from build123d import *

# Parameters (mm, degrees)
F1_DEPTH       = 25
F2_DEPTH       = 10
F3_DEPTH       = 30
F4_DEPTH       = 20
F5_DEPTH       = 10
F7_D           = 14.75
F7_CBORE_D     = 22.25
F7_CBORE_DEPTH = 14
F8_SIZE        = 5
F9_R           = 7.49999


# Not quite as in the source:
# - a fillet or chamfer is up to 0.001 mm smaller than in the source, because OpenCascade refuses the exact size


with BuildPart() as f1:
    # F0 (on Front) → F1 (new body)
    with BuildSketch(Plane.XZ):
        with BuildLine():
            Line((96.5, 100), (-96.5, 100))
            ThreePointArc((-96.5, 100), (-103.5710678119, 97.0710678119), (-106.5, 90))
            Line((-106.5, 90), (-106.5, -90))
            ThreePointArc((-106.5, -90), (-103.5710678119, -97.0710678119), (-96.5, -100))
            Line((-96.5, -100), (-63.5, -100))
            Line((-63.5, -100), (-63.5, -42.2497216032))
            ThreePointArc((-63.5, -42.2497216032), (-58.0047374401, -26.6111405489), (-43.9347826087, -17.8476082112))
            ThreePointArc((-43.9347826087, -17.8476082112), (0.1396103068, 6.3603896932), (24.3476082112, 50.4347826087))
            ThreePointArc((24.3476082112, 50.4347826087), (33.1111405489, 64.5047374401), (48.7497216032, 70))
            Line((48.7497216032, 70), (106.5, 70))
            Line((106.5, 70), (106.5, 90))
            ThreePointArc((106.5, 90), (103.5710678119, 97.0710678119), (96.5, 100))
        make_face()
        with BuildLine():
            ThreePointArc((17.5, 70), (-6.2243507239, 12.7243507239), (-63.5, -11))
            Line((-63.5, -11), (-87.5, -11))
            ThreePointArc((-87.5, -11), (-94.5710678119, -8.0710678119), (-97.5, -1))
            Line((-97.5, -1), (-97.5, 81))
            ThreePointArc((-97.5, 81), (-94.5710678119, 88.0710678119), (-87.5, 91))
            Line((-87.5, 91), (7.5, 91))
            ThreePointArc((7.5, 91), (14.5710678119, 88.0710678119), (17.5, 81))
            Line((17.5, 81), (17.5, 70))
        make_face(mode=Mode.SUBTRACT)
        with BuildLine():
            Line((106.5, 55), (106.5, 70))
            Line((106.5, 70), (48.7497216032, 70))
            ThreePointArc((48.7497216032, 70), (33.1111405489, 64.5047374401), (24.3476082112, 50.4347826087))
            ThreePointArc((24.3476082112, 50.4347826087), (0.1396103068, 6.3603896932), (-43.9347826087, -17.8476082112))
            ThreePointArc((-43.9347826087, -17.8476082112), (-58.0047374401, -26.6111405489), (-63.5, -42.2497216032))
            Line((-63.5, -42.2497216032), (-63.5, -100))
            Line((-63.5, -100), (-48.5, -100))
            Line((-48.5, -100), (-48.5, -42.2497216032))
            ThreePointArc((-48.5, -42.2497216032), (-46.3018949761, -35.9942891815), (-40.6739130435, -32.4888762464))
            ThreePointArc((-40.6739130435, -32.4888762464), (10.7462120246, -4.2462120246), (38.9888762464, 47.1739130435))
            ThreePointArc((38.9888762464, 47.1739130435), (42.4942891815, 52.8018949761), (48.7497216032, 55))
            Line((48.7497216032, 55), (106.5, 55))
        make_face()
        with BuildLine():
            Line((106.5, -40), (106.5, 55))
            Line((106.5, 55), (48.7497216032, 55))
            ThreePointArc((48.7497216032, 55), (42.4942891815, 52.8018949761), (38.9888762464, 47.1739130435))
            ThreePointArc((38.9888762464, 47.1739130435), (10.7462120246, -4.2462120246), (-40.6739130435, -32.4888762464))
            ThreePointArc((-40.6739130435, -32.4888762464), (-46.3018949761, -35.9942891815), (-48.5, -42.2497216032))
            Line((-48.5, -42.2497216032), (-48.5, -100))
            Line((-48.5, -100), (46.5, -100))
            Line((46.5, -100), (46.5, -55))
            ThreePointArc((46.5, -55), (50.8933982822, -44.3933982822), (61.5, -40))
            Line((61.5, -40), (106.5, -40))
        make_face()
        with BuildLine():
            ThreePointArc((46.130896205, 38.7419354839), (49.7234965193, 43.981834214), (55.7476414861, 46))
            Line((55.7476414861, 46), (87.5, 46))
            ThreePointArc((87.5, 46), (94.5710678119, 43.0710678119), (97.5, 36))
            Line((97.5, 36), (97.5, -21))
            ThreePointArc((97.5, -21), (94.5710678119, -28.0710678119), (87.5, -31))
            Line((87.5, -31), (61.5, -31))
            ThreePointArc((61.5, -31), (44.5294372515, -38.0294372515), (37.5, -55))
            Line((37.5, -55), (37.5, -81))
            ThreePointArc((37.5, -81), (34.5710678119, -88.0710678119), (27.5, -91))
            Line((27.5, -91), (-29.5, -91))
            ThreePointArc((-29.5, -91), (-36.5710678119, -88.0710678119), (-39.5, -81))
            Line((-39.5, -81), (-39.5, -49.2476414861))
            ThreePointArc((-39.5, -49.2476414861), (-37.481834214, -43.2234965193), (-32.2419354839, -39.630896205))
            ThreePointArc((-32.2419354839, -39.630896205), (17.1101730553, -10.6101730553), (46.130896205, 38.7419354839))
        make_face(mode=Mode.SUBTRACT)
        with BuildLine():
            Line((106.5, -90), (106.5, -40))
            Line((106.5, -40), (61.5, -40))
            ThreePointArc((61.5, -40), (50.8933982822, -44.3933982822), (46.5, -55))
            Line((46.5, -55), (46.5, -100))
            Line((46.5, -100), (96.5, -100))
            ThreePointArc((96.5, -100), (103.5710678119, -97.0710678119), (106.5, -90))
        make_face()
        with BuildLine():
            Line((-87.5, -11), (-63.5, -11))
            ThreePointArc((-63.5, -11), (-6.2243507239, 12.7243507239), (17.5, 70))
            Line((17.5, 70), (17.5, 81))
            ThreePointArc((17.5, 81), (14.5710678119, 88.0710678119), (7.5, 91))
            Line((7.5, 91), (-87.5, 91))
            ThreePointArc((-87.5, 91), (-94.5710678119, 88.0710678119), (-97.5, 81))
            Line((-97.5, 81), (-97.5, -1))
            ThreePointArc((-97.5, -1), (-94.5710678119, -8.0710678119), (-87.5, -11))
        make_face()
        with BuildLine():
            Line((87.5, 46), (55.7476414861, 46))
            ThreePointArc((55.7476414861, 46), (49.7234965193, 43.981834214), (46.130896205, 38.7419354839))
            ThreePointArc((46.130896205, 38.7419354839), (17.1101730553, -10.6101730553), (-32.2419354839, -39.630896205))
            ThreePointArc((-32.2419354839, -39.630896205), (-37.481834214, -43.2234965193), (-39.5, -49.2476414861))
            Line((-39.5, -49.2476414861), (-39.5, -81))
            ThreePointArc((-39.5, -81), (-36.5710678119, -88.0710678119), (-29.5, -91))
            Line((-29.5, -91), (27.5, -91))
            ThreePointArc((27.5, -91), (34.5710678119, -88.0710678119), (37.5, -81))
            Line((37.5, -81), (37.5, -55))
            ThreePointArc((37.5, -55), (44.5294372515, -38.0294372515), (61.5, -31))
            Line((61.5, -31), (87.5, -31))
            ThreePointArc((87.5, -31), (94.5710678119, -28.0710678119), (97.5, -21))
            Line((97.5, -21), (97.5, 36))
            ThreePointArc((97.5, 36), (94.5710678119, 43.0710678119), (87.5, 46))
        make_face()
    extrude(amount=-F1_DEPTH)

    # F0 (on Front) → F2 (join)
    with BuildSketch(Plane.XZ):
        with BuildLine():
            Line((-87.5, -11), (-63.5, -11))
            ThreePointArc((-63.5, -11), (-6.2243507239, 12.7243507239), (17.5, 70))
            Line((17.5, 70), (17.5, 81))
            ThreePointArc((17.5, 81), (14.5710678119, 88.0710678119), (7.5, 91))
            Line((7.5, 91), (-87.5, 91))
            ThreePointArc((-87.5, 91), (-94.5710678119, 88.0710678119), (-97.5, 81))
            Line((-97.5, 81), (-97.5, -1))
            ThreePointArc((-97.5, -1), (-94.5710678119, -8.0710678119), (-87.5, -11))
        make_face()
    extrude(amount=F2_DEPTH)

    # F0 (on Front) → F3 (join)
    with BuildSketch(Plane.XZ):
        with BuildLine():
            Line((106.5, 55), (106.5, 70))
            Line((106.5, 70), (48.7497216032, 70))
            ThreePointArc((48.7497216032, 70), (33.1111405489, 64.5047374401), (24.3476082112, 50.4347826087))
            ThreePointArc((24.3476082112, 50.4347826087), (0.1396103068, 6.3603896932), (-43.9347826087, -17.8476082112))
            ThreePointArc((-43.9347826087, -17.8476082112), (-58.0047374401, -26.6111405489), (-63.5, -42.2497216032))
            Line((-63.5, -42.2497216032), (-63.5, -100))
            Line((-63.5, -100), (-48.5, -100))
            Line((-48.5, -100), (-48.5, -42.2497216032))
            ThreePointArc((-48.5, -42.2497216032), (-46.3018949761, -35.9942891815), (-40.6739130435, -32.4888762464))
            ThreePointArc((-40.6739130435, -32.4888762464), (10.7462120246, -4.2462120246), (38.9888762464, 47.1739130435))
            ThreePointArc((38.9888762464, 47.1739130435), (42.4942891815, 52.8018949761), (48.7497216032, 55))
            Line((48.7497216032, 55), (106.5, 55))
        make_face()
    extrude(amount=F3_DEPTH)

    # F0 (on Front) → F4 (cut)
    with BuildSketch(Plane.XZ):
        with BuildLine():
            Line((87.5, 46), (55.7476414861, 46))
            ThreePointArc((55.7476414861, 46), (49.7234965193, 43.981834214), (46.130896205, 38.7419354839))
            ThreePointArc((46.130896205, 38.7419354839), (17.1101730553, -10.6101730553), (-32.2419354839, -39.630896205))
            ThreePointArc((-32.2419354839, -39.630896205), (-37.481834214, -43.2234965193), (-39.5, -49.2476414861))
            Line((-39.5, -49.2476414861), (-39.5, -81))
            ThreePointArc((-39.5, -81), (-36.5710678119, -88.0710678119), (-29.5, -91))
            Line((-29.5, -91), (27.5, -91))
            ThreePointArc((27.5, -91), (34.5710678119, -88.0710678119), (37.5, -81))
            Line((37.5, -81), (37.5, -55))
            ThreePointArc((37.5, -55), (44.5294372515, -38.0294372515), (61.5, -31))
            Line((61.5, -31), (87.5, -31))
            ThreePointArc((87.5, -31), (94.5710678119, -28.0710678119), (97.5, -21))
            Line((97.5, -21), (97.5, 36))
            ThreePointArc((97.5, 36), (94.5710678119, 43.0710678119), (87.5, 46))
        make_face()
    extrude(amount=-F4_DEPTH, mode=Mode.SUBTRACT)

    # F0 (on Front) → F5 (join)
    with BuildSketch(Plane.XZ):
        with BuildLine():
            Line((106.5, -90), (106.5, -40))
            Line((106.5, -40), (61.5, -40))
            ThreePointArc((61.5, -40), (50.8933982822, -44.3933982822), (46.5, -55))
            Line((46.5, -55), (46.5, -100))
            Line((46.5, -100), (96.5, -100))
            ThreePointArc((96.5, -100), (103.5710678119, -97.0710678119), (106.5, -90))
        make_face()
    extrude(amount=F5_DEPTH)

    # F7 (through all)
    with Locations(Plane.XZ.offset(10)):
        with Locations((77.2273465991, -70.3643187881)):
            CounterBoreHole(F7_D / 2, F7_CBORE_D / 2, F7_CBORE_DEPTH)

    # F8
    f8_edges = [f1.edges().sort_by_distance(p)[0] for p in [
        (-97.5, -10, 40),
    ]]
    chamfer(f8_edges, length=F8_SIZE)

    # F9 (radius 7.5 in the source; OpenCascade refuses exactly that, so slightly less here)
    f9_edges = [f1.edges().sort_by_distance(p)[0] for p in [
        (-63.5, -30, -71.124861),
        (-48.5, -30, -71.124861),
    ]]
    fillet(f9_edges, radius=F9_R)


solid = f1.part
CAD build for the part. Positions are in the model's coordinates, mm. A direction names the side the tool comes from. Round coordinates to 2 decimals unless told otherwise and drop trailing zeros. Order: outer loops, then holes, each group sorted by start corner. A loop starts at its lowest first (then second) coordinate and runs counter-clockwise, first axis right, second up. Notation, with made-up numbers: (85.25, -10.5) - (121.25, -10.5) arc R25 ccw to (121.25, 3.5) - close; hole circle Ø6 at (26, 10.25). An arc over 180 degrees is marked (long way). Return JSON: item names as keys, results as strings.
(1) Wall check: probe 1 along Z at (x, y) = (21.5, 1); probe 2 along Z at (x, y) = (91.5, -3.5); probe 3 along X at (y, z) = (-10.5, -68.5). Give the ranges that are in metal, low to high. Write a range as from..to.
Answer key:
{"probe 1": "z = -100..-91, -5.97..100", "probe 2": "z = -100..-40, 55..70", "probe 3": "x = -63.5..-48.5"}
(2) Cut at C-C (y = -2.5). Give the cut face in (x, z) (3 decimals), then the cut area to 3 significant figures.
Answer key:
{"outline": "(-97.5, -1) arc R10 ccw to (-87.5, -11) - (-63.5, -11) arc R81 ccw to (17.5, 70) - (17.5, 81) arc R10 ccw to (7.5, 91) - (-87.5, 91) arc R10 ccw to (-97.5, 81) - close; (-63.5, -100) - (-48.5, -100) - (-48.5, -42.25) arc R10 cw to (-40.674, -32.489) arc R105 ccw to (38.989, 47.174) arc R10 cw to (48.75, 55) - (106.5, 55) - (106.5, 70) - (48.75, 70) arc R25 ccw to (24.348, 50.435) arc R90 cw to (-43.935, -17.848) arc R25 ccw to (-63.5, -42.25) - close; (46.5, -100) - (96.5, -100) arc R10 ccw to (106.5, -90) - (106.5, -40) - (61.5, -40) arc R15 ccw to (46.5, -55) - close; hole circle Ø22.25 at (77.227, -70.364)", "area": "17,500 mm^2"}
(3) Cut at A-A (x = -67). Give the cut face in (y, z).
Answer key:
{"outline": "(-10, -6) - (-5, -11) - (0, -11) - (0, -100) - (25, -100) - (25, 100) - (0, 100) - (0, 91) - (-5, 91) - (-10, 86) - close"}
(4) Pin check, flat tips, straight feed: pin 1 Ø5.5 at (y, z) = (-3, 43) entering from -X; pin 2 Ø6 at (x, z) = (49.5, 24) entering from -Y; pin 3 Ø1.5 at (x, y) = (-79, -1.5) entering from -Z. Stop position of each tip, or through.
Answer key:
{"pin 1": "stops at x = -97.5", "pin 2": "stops at y = 20", "pin 3": "stops at z = -11"}
(5) Tool access for faces 1 (the face through (78.029, -27.861, 57.255)), 2 (the face through (-6.858, -2.465, 12.098)), 3 (the face through (-48.5, -11, -72)): list every direction of +Z, -Z, +X, -X, +Y, -Y with a clear straight run to the whole face (end or side of a thin tool).
Answer key:
{"face 1": "-Z, +X, -Y", "face 2": "-Y", "face 3": "-Z, -Y"}
(6) Cut at D-D (y = 10). Give the cut face in (x, z) (3 decimals), then the cut area to 3 significant figures.
Answer key:
{"outline": "(-106.5, -90) arc R10 ccw to (-96.5, -100) - (96.5, -100) arc R10 ccw to (106.5, -90) - (106.5, 90) arc R10 ccw to (96.5, 100) - (-96.5, 100) arc R10 ccw to (-106.5, 90) - close; hole (-39.5, -81) arc R10 ccw to (-29.5, -91) - (27.5, -91) arc R10 ccw to (37.5, -81) - (37.5, -55) arc R24 cw to (61.5, -31) - (87.5, -31) arc R10 ccw to (97.5, -21) - (97.5, 36) arc R10 ccw to (87.5, 46) - (55.748, 46) arc R10 ccw to (46.131, 38.742) arc R114 cw to (-32.242, -39.631) arc R10 ccw to (-39.5, -49.248) - close; hole circle Ø14.75 at (77.227, -70.364)", "area": "32,500 mm^2"}
(7) Pull direction X, two halves, no side cores. Call faces 4 (the face through (-39, -8, 88)), 5 (the face through (17.681, 9.86, -10.035)), 6 (the face through (-61.361, -27.745, -71.529)), 7 (the face through (68.399, -3.098, -77.134)): +X half, -X half, draft (parallel to the pull), parting line (faces both ways), or undercut.
Answer key:
{"face 4": "draft", "face 5": "undercut", "face 6": "-X half", "face 7": "undercut"}
